The model under review builds one solid part; all positions refer to its coordinate system, in mm. A direction names the side the tool comes from. Give positions to 0.01 mm unless a question says otherwise; leave off trailing zeros. Loops run counter-clockwise (first coordinate to the right, second up) from the corner with the lowest first, then second, coordinate; pieces in that order, holes last. Notation, with made-up numbers: M -1.5,-16.5 L 9.5,-16.5 A28 ccw 9.5,3.5 Z; hole C -22,84.5 d7. An arc over 180 degrees is marked long. Return JSON: item names as keys, results as strings.
```python
from build123d import *

# Parameters (mm, degrees)
ESQUISSE1_R        = 500
BOSS_EXTRU_1_DEPTH = 100
ESQUISSE2_W        = 200
ESQUISSE2_H        = 200
BOSS_EXTRU_2_DEPTH = 1000
ESQUISSE3_R        = 50
BOSS_EXTRU_3_DEPTH = 95
CONG_1_R           = 50
CONG_2_R           = 20
CONG_3_R           = 20


with BuildPart() as part:
    # Esquisse1 → Boss.-Extru.1 (new body)
    with BuildSketch(Plane(origin=(0, 0, 0), x_dir=(0, 0, -1), z_dir=(1, 0, 0))):
        Circle(ESQUISSE1_R)
    extrude(amount=BOSS_EXTRU_1_DEPTH)

    # Esquisse2 → Boss.-Extru.2 (add)
    with BuildSketch(Plane(origin=(100, 0, 0), x_dir=(0, 0, -1), z_dir=(1, 0, 0))):
        Rectangle(ESQUISSE2_W, ESQUISSE2_H)
    extrude(amount=BOSS_EXTRU_2_DEPTH)

    # Esquisse3 → Boss.-Extru.3 (add)
    with BuildSketch(Plane(origin=(1100, 0, 0), x_dir=(0, 0, -1), z_dir=(1, 0, 0))):
        Circle(ESQUISSE3_R)
    extrude(amount=BOSS_EXTRU_3_DEPTH)

    # Congé1
    cong_1_edges = [part.edges().sort_by_distance(p)[0] for p in [
        (100, 0, 500),
    ]]
    fillet(cong_1_edges, radius=CONG_1_R)

    # Congé2
    cong_2_edges = [part.edges().sort_by_distance(p)[0] for p in [
        (600, -100, -100),
        (600, 100, -100),
        (600, 100, 100),
        (600, -100, 100),
    ]]
    fillet(cong_2_edges, radius=CONG_2_R)

    # Congé3
    cong_3_edges = [part.edges().sort_by_distance(p)[0] for p in [
        (1100, 100, 0),
        (1100, 0, -100),
        (1100, 0, 100),
        (1100, -100, 0),
        (1100, 94.142135624, 94.142135624),
        (1100, -94.142135624, 94.142135624),
        (1100, -94.142135624, -94.142135624),
        (1100, 94.142135624, -94.142135624),
    ]]
    fillet(cong_3_edges, radius=CONG_3_R)


solid = part.part
```
1) Consider section B-B on x = 379. Write out the cut boundary in (y, z), then the cut area to 3 significant figures.
From the geometry:
{"outline": "M -100,-80 A20 ccw -80,-100 L 80,-100 A20 ccw 100,-80 L 100,80 A20 ccw 80,100 L -80,100 A20 ccw -100,80 Z", "area": "39,700 mm²"}
2) Tool access review of faces 1 (the face through (583, -100, 1)), 2 (the face through (583, 100, 1)), 3 (the face through (583, -1, 100)), 4 (the face through (583, -1, -100)), 5 (the face through (1100, 37, 37)): name each direction out of +Z, -Z, +X, -X, +Y, -Y from which nothing blocks a thin tool from reaching the whole face with its end or side.
From the geometry:
{"face 1": "+Z, -Z, +X, -Y", "face 2": "+Z, -Z, +X, +Y", "face 3": "+Z, +X, +Y, -Y", "face 4": "-Z, +X, +Y, -Y", "face 5": "+X"}
3) Wall thickness on L1, parallel to X at y = 345.5, z = 8; L2, parallel to Y at x = 170, z = 83.5; L3, parallel to Y at x = 745, z = 58: over which ranges is each line inside the solid? List them lowest first. Write a range as from..to.
From the geometry:
{"L1": "0..100", "L2": "-99.69..99.69", "L3": "-100..100"}
4) Insertion check: pin 1 (10 mm diameter, centred on y = 198, z = -287, fed in from -X); pin 2 (3 mm diameter, centred on x = 370, z = -87.5, fed in from -Y). Each pin has a flat end and moves straight along its axis. Give the tip position at first contact, or say it passes through.
From the geometry:
{"pin 1": "x = 0", "pin 2": "y = -99.08"}
5) Consider section A-A on y = 0. Write out the cut boundary in (x, z).
From the geometry:
{"outline": "M 0,-500 L 50,-500 A50 ccw 100,-450 L 100,-100 L 1080,-100 A20 ccw 1100,-80 L 1100,-50 L 1195,-50 L 1195,50 L 1100,50 L 1100,80 A20 ccw 1080,100 L 100,100 L 100,450 A50 ccw 50,500 L 0,500 Z"}
